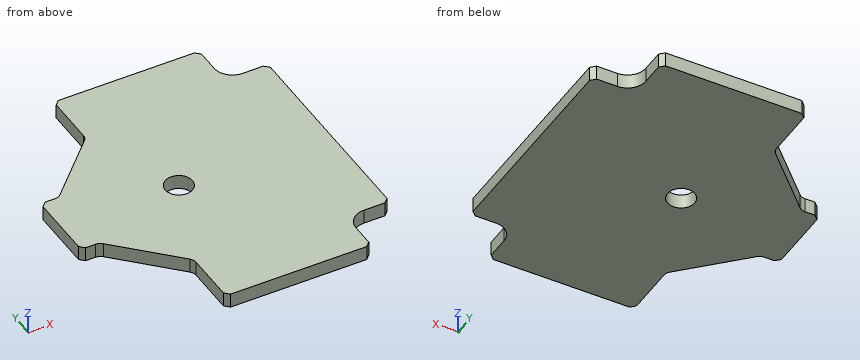
Autodesk Inventor part; units mm, degrees
ref_plane "YZ Plane" through (0, 0, 0) normal (1, 0, 0) x (0, 1, 0)
ref_plane "XZ Plane" through (0, 0, 0) normal (0, 1, 0) x (-1, 0, 0)
ref_plane "XY Plane" through (0, 0, 0) normal (0, 0, 1) x (1, 0, 0)
sketch "スケッチ1" plane through (0, 0, 0) normal (0, 0, 1) x (1, 0, 0)
  line L0 (16.5, 0) -> (16.5, 11.5)
  line L1 (11.2044, 17) -> (-3.7956, 17)
  line L2 (-3.7956, 17) -> (-4.2956, 16.5)
  line L3 (-4.2956, 16.5) -> (-4.2956, 11.1093)
  arc A0 (-4.5885, 10.4022) -> (-4.2956, 11.1093) centre (-5.2956, 11.1093) ccw
  line L4 (-4.5885, 10.4022) -> (-10.6978, 4.2929)
  arc A1 (-11.4049, 4) -> (-10.6978, 4.2929) centre (-11.4049, 5) ccw
  line L5 (-11.4049, 4) -> (-12.5, 4)
  line L6 (-12.5, 4) -> (-13, 3.5)
  line L7 (-13, 3.5) -> (-13, 0)
  circle A2 centre (0, 0) radius 1.5
  line L8 (16, 12) -> (13.7044, 12)
  line L9 (11.7044, 14) -> (11.7044, 16.5)
  line L10 (16.5, 11.5) -> (16, 12)
  line L11 (11.7044, 16.5) -> (11.2044, 17)
  line L12 (0, 0) -> (16.5, 0) construction
  arc A3 (11.7044, 14) -> (13.7044, 12) centre (13.7044, 14) ccw
  line L13 (11.7044, 17) -> (11.7044, 18.5) construction
  line L14 (0, 0) -> (-13, 0) construction
  line L15 (-13, -2) -> (-13, 2) construction
  line L16 (-10.6978, 4.2929) -> (-5.2974, 9.6932) construction
  line L17 (-4.2956, 17) -> (-4.2956, 11.1093) construction
  line L18 (16.5, 0) -> (16.5, -11.5)
  line L19 (11.2044, -17) -> (-3.7956, -17)
  line L20 (-3.7956, -17) -> (-4.2956, -16.5)
  line L21 (-4.2956, -16.5) -> (-4.2956, -11.1093)
  arc A4 (-4.2956, -11.1093) -> (-4.5885, -10.4022) centre (-5.2956, -11.1093) ccw
  line L22 (-4.5885, -10.4022) -> (-10.6978, -4.2929)
  arc A5 (-10.6978, -4.2929) -> (-11.4049, -4) centre (-11.4049, -5) ccw
  line L23 (-11.4049, -4) -> (-12.5, -4)
  line L24 (-12.5, -4) -> (-13, -3.5)
  line L25 (-13, -3.5) -> (-13, 0)
  line L26 (16, -12) -> (13.7044, -12)
  line L27 (11.7044, -14) -> (11.7044, -16.5)
  line L28 (16.5, -11.5) -> (16, -12)
  line L29 (11.7044, -16.5) -> (11.2044, -17)
  arc A6 (13.7044, -12) -> (11.7044, -14) centre (13.7044, -14) ccw
  dimension "d5" = 0.5
  dimension "d6" = 0.5
  dimension "d7" = 16.5
  dimension "d8" = 2
  dimension "d9" = 12
  dimension "d10" = 17
  dimension "d11" = 0.5
  dimension "d12" = 0.5
  dimension "d14" = 0.5
  dimension "d15" = 0.5
  dimension "d16" = 4
  dimension "d18" = 0.5
  dimension "d19" = 0.5
  dimension "d20" = 1
  dimension "d21" = 3
extrude "押し出し1" add sketch "スケッチ1" along normal blind 1.6
properties part number "force_sensor_pcb"
Input: part model. Units: mm. Frame: model coordinates. Give positions to 0.01 mm unless a question says otherwise; leave off trailing zeros. Order: outer loops, then holes, each group sorted by start corner. A loop starts at its lowest first (then second) coordinate and runs counter-clockwise, first axis right, second up. Notation, with made-up numbers: (24, 70.5) -> (53, 70.5) arc R35 ccw to (53, 105.5) -> close; hole circle Ø3 at (41, 63). An arc over 180 degrees is marked (long way). Use one line per item in the form item = value.
1) Line query: probe 1 along Y at (x, z) = (0, 0.7); probe 2 along X at (y, z) = (-14.5, 1); probe 3 along X at (y, z) = (-11.5, 1). Output: solid intervals per line, ascending.
Response values:
probe_1 = -17 to -1.5, 1.5 to 17
probe_2 = -4.3 to 11.7
probe_3 = -4.3 to 16.5
2) First-contact query: pin 1 Ø0.8 at (y, z) = (-14, 0.5) entering from -X; pin 2 Ø0.5 at (y, z) = (-15, 1) entering from +X; pin 3 Ø0.9 at (x, z) = (-12, 0.5) entering from -Y. Flat tips, straight axial feed; report the tip coordinate or a pass-through.
Response values:
pin_1 = -4.3
pin_2 = 11.7
pin_3 = -4
3) Section D-D, the plane x = 14.25. Return loops of the section in (y, z), and give its area (3 significant figures).
Response values:
outline = (-12, 0) -> (12, 0) -> (12, 1.6) -> (-12, 1.6) -> close
area = 38.4 mm^2
4) Section C-C, the plane x = 0. Return loops of the section in (y, z).
Response values:
outline = (-17, 0) -> (-1.5, 0) -> (-1.5, 1.6) -> (-17, 1.6) -> close; (1.5, 0) -> (17, 0) -> (17, 1.6) -> (1.5, 1.6) -> close
5) Section A-A, the plane y = 0. Return loops of the section in (x, z), and give its area (3 significant figures).
Response values:
outline = (-13, 0) -> (-1.5, 0) -> (-1.5, 1.6) -> (-13, 1.6) -> close; (1.5, 0) -> (16.5, 0) -> (16.5, 1.6) -> (1.5, 1.6) -> close
area = 42.4 mm^2
